from build123d import *


with BuildPart() as part:
    # Sketch1 → Revolve1 (revolve)
    with BuildSketch(Plane.XY):
        with BuildLine():
            Line((6, 12), (-6, 12))
            Line((-6, 12), (-6, 9.33862945))
            ThreePointArc((-6, 9.33862945), (-5.025719768, 9.897077388), (-4, 10.35422619))
            Line((-4, 10.35422619), (-4, 10.675204916))
            ThreePointArc((-4, 10.675204916), (0, 11.4), (4, 10.675204916))
            Line((4, 10.675204916), (4, 10.35422619))
            ThreePointArc((4, 10.35422619), (5.025719768, 9.897077388), (6, 9.33862945))
            Line((6, 9.33862945), (6, 12))
        make_face()
    revolve(axis=Axis((48.348883339, 0, 0), (-1, 0, 0)))


solid = part.part
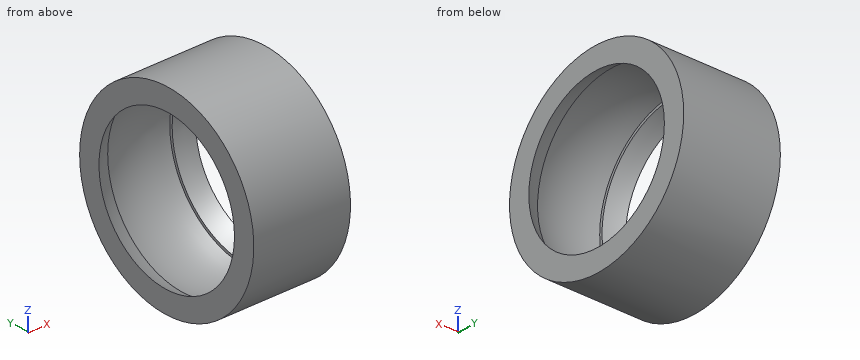
Read the model definition and answer for the solid it produces. Units are mm, in the model's axes. Round coordinates to 2 decimals unless told otherwise and drop trailing zeros. Order: outer loops, then holes, each group sorted by start corner. A loop starts at its lowest first (then second) coordinate and runs counter-clockwise, first axis right, second up.
1) Flat-ended cylindrical pins translate along their axes: pin 1 (4 mm diameter, centred on x = 0, z = 3.5, fed in from +Y); pin 2 (2 mm diameter, centred on x = 2, z = 5.5, fed in from -Y); pin 3 (1.5 mm diameter, centred on x = 2, z = 9, fed in from +Y). Find the tip coordinate at first contact, or state that the pin passes through.
2) The part is cut by section D-D on x = -4.5. Write down the section's boundary in (y, z).
3) The part is cut by section B-B on y = 0. Write down the section's boundary in (x, z).
4) The part is cut by section C-C on z = 10. Write down the section's boundary in (x, y), plus the area to 3 significant figures.
5) The part is cut by section A-A on z = -9. Write down the section's boundary in (x, y), plus the area to 3 significant figures.
6) Straight lines are drawn through the part: L1, parallel to X at y = -10, z = 0.25; L2, parallel to Z at x = -2, y = 3; L3, parallel to Y at x = 0.25, z = 5.75. For each, find the intervals that lie inside material, in ascending order.
Resolved:
1. pin 1: stops at y = 11.91
1. pin 2: stops at y = -11.12
1. pin 3: stops at y = 8.71
2. outline: circle Ø24 at (0, 0); hole circle Ø20.29 at (0, 0)
3. outline: (-6, -12) - (6, -12) - (6, -9.34) arc R11.1 cw to (4, -10.35) - (4, -10.68) arc R11.4 cw to (-4, -10.68) - (-4, -10.35) arc R11.1 cw to (-6, -9.34) - close; (-6, 9.34) arc R11.1 cw to (-4, 10.35) - (-4, 10.68) arc R11.4 cw to (4, 10.68) - (4, 10.35) arc R11.1 cw to (6, 9.34) - (6, 12) - (-6, 12) - close
4. outline: (-6, -6.63) - (6, -6.63) - (6, 6.63) - (-6, 6.63) - close; hole (-4, -3.74) arc R5.47 ccw to (4, -3.74) - (4, -2.69) arc R4.82 ccw to (4, 2.69) - (4, 3.74) arc R5.47 ccw to (-4, 3.74) - (-4, 2.69) arc R4.82 ccw to (-4, -2.69) - close
4. area: 74.2 mm2
5. outline: (-6, -7.94) - (6, -7.94) - (6, -2.49) arc R6.5 cw to (4, -5.12) - (4, -5.74) arc R7 cw to (-4, -5.74) - (-4, -5.12) arc R6.5 cw to (-6, -2.49) - close; (-6, 2.49) arc R6.5 cw to (-4, 5.12) - (-4, 5.74) arc R7 cw to (4, 5.74) - (4, 5.12) arc R6.5 cw to (6, 2.49) - (6, 7.94) - (-6, 7.94) - close
5. area: 52.6 mm2
6. L1: x = -6 to -4.81, 4.81 to 6
6. L2: z = -11.62 to -10.81, 10.81 to 11.62
6. L3: y = -10.53 to -9.84, 9.84 to 10.53
